Could you check a few things on this model? Use its own coordinates, in mm. A direction names the side the tool comes from. Round coordinates to 2 decimals unless told otherwise and drop trailing zeros. Write each loop counter-clockwise with the first axis right and the second up, starting at its lowest first coordinate (ties: lowest second). Pieces come first, ordered by that corner, then holes. Notation, with made-up numbers: M 63.25,28 L 116.25,28 A12 ccw 116.25,38 Z; hole C 63,78 d9. An arc over 180 degrees is marked long. One line per question, with ' | ' between items. Start each with the question number.
```python
from build123d import *

# Parameters (mm, degrees)
ESBO_O1_W                = 29
ESBO_O1_H                = 19
ESBO_O1_R                = 1.25
RESSALTO_EXTRUS_O1_DEPTH = 2
ESBO_O2_R                = 4
ESBO_O2_R_2              = 1.25
RESSALTO_EXTRUS_O2_DEPTH = 2


with BuildPart() as part:
    # Esboço1 → Ressalto-extrusão1 (new body)
    with BuildSketch(Plane(origin=(0, 0, 0), x_dir=(0, 0, -1), z_dir=(1, 0, 0))):
        with Locations((2.073076923, -0.498076923)):
            Rectangle(ESBO_O1_W, ESBO_O1_H)
        with Locations((8.073076923, 0.001923077)):
            Circle(ESBO_O1_R, mode=Mode.SUBTRACT)
        with Locations((-5.926923077, 0.001923077)):
            Circle(ESBO_O1_R, mode=Mode.SUBTRACT)
    extrude(amount=RESSALTO_EXTRUS_O1_DEPTH)

    # Esboço2 → Ressalto-extrusão2 (add)
    # profile 1 of 2: a face of its own
    with BuildSketch(Plane(origin=(2, 0, 0), x_dir=(0, 0, -1), z_dir=(1, 0, 0))):
        with Locations((8.073076923, 0)):
            Circle(ESBO_O2_R)
        with Locations(Location((8.073076923, 0, 0), (0, 0, 179.955926319))):
            Circle(ESBO_O2_R_2, mode=Mode.SUBTRACT)
    # profile 2 of 2: a face of its own
    with BuildSketch(Plane(origin=(2, 0, 0), x_dir=(0, 0, -1), z_dir=(1, 0, 0))):
        with Locations((-5.926923077, 0)):
            Circle(ESBO_O2_R)
        with Locations(Location((-5.926923077, 0, 0), (0, 0, 179.955926319))):
            Circle(ESBO_O2_R_2, mode=Mode.SUBTRACT)
    extrude(amount=RESSALTO_EXTRUS_O2_DEPTH)


solid = part.part
```
1. Suppose I cut it at D-D (z = 3.75). Write out the boundary of the cut face in (x, y), and give its area (3 significant figures).
2. I need wall thicknesses on line 1 along X through (y, z) = (-1.5, -14); line 2 along Z through (x, y) = (2.95, 3.5); line 3 along Z through (x, y) = (2.5, 3). Which ranges of each line are inside material? Lowest first, please. Write a range as from..to.
3. Suppose I cut it at B-B (y = 4.75). Write out the boundary of the cut face in (x, z), and give its area (3 significant figures).
4. I'm going to push flat-ended pins straight in: P1, Ø1, axis at y = 3.5, z = -3.5, coming from the +X side; P2, Ø1, axis at y = -0.5, z = 6, coming from the +X side. Where does each tip first touch, or does it pass through?
5. Suppose I cut it at C-C (x = 1.5). Write out the boundary of the cut face in (y, z), and give its area (3 significant figures).
6. Which directions (+Z, -Z, +X, -X, +Y, -Y) give clear straight access to the entire face, cutting with the end or side of a thin tool? Please do faces 1 (the face through (2, 0, -2)), 2 (the face through (1, -1, -16.573)).
Computed:
1) outline: M 0,-10 L 2,-10 L 2,-3.36 L 4,-3.36 L 4,3.36 L 2,3.36 L 2,9 L 0,9 Z | area: 51.4 mm²
2) line 1: x = 0..2 | line 2: z = -10.01..-6.14, 3.99..7.86 | line 3: z = -10.72..-5.43, 3.28..8.57
3) outline: M 0,-16.57 L 2,-16.57 L 2,12.43 L 0,12.43 Z | area: 58.0 mm²
4) P1: stops at x = 2 | P2: passes through
5) outline: M -10,-16.57 L 9,-16.57 L 9,12.43 L -10,12.43 Z; hole C 0,-8.07 d2.5; hole C 0,5.93 d2.5 | area: 541 mm²
6) face 1: +X | face 2: -Z, +X, -X, +Y, -Y
